from build123d import *

# Parameters (mm, degrees)
BASE_SKETCH_W           = 585.98
BASE_SKETCH_H           = 191.39
BOSS_EXTRUDE1_DEPTH     = 11.81
JOINT_X_W               = 25.4
JOINT_X_H               = 11.81
BOSS_EXTRUDE2_DEPTH     = 11.81
LPATTERN1_COUNT         = 4
LPATTERN1_PITCH         = 186.86
JOINT_Y_W               = 11.81
JOINT_Y_H               = 25.4
BOSS_EXTRUDE3_DEPTH     = 11.81
LPATTERN2_COUNT         = 4
LPATTERN2_PITCH         = 59.266666667
MIRROR3_COPY_1_SKETCH_W = 11.81
MIRROR3_COPY_1_SKETCH_H = 25.4
MIRROR3_COPY_1_DEPTH    = 11.81
MIRROR3_COPY_2_SKETCH_W = 11.81
MIRROR3_COPY_2_SKETCH_H = 25.4
MIRROR3_COPY_2_DEPTH    = 11.81
MIRROR3_COPY_3_SKETCH_W = 11.81
MIRROR3_COPY_3_SKETCH_H = 25.4
MIRROR3_COPY_3_DEPTH    = 11.81


with BuildPart() as part:
    # Base_Sketch → Boss-Extrude1 (new body)
    with BuildSketch(Plane.XY):
        with Locations((0, -4.040082085)):
            Rectangle(BASE_SKETCH_W, BASE_SKETCH_H)
    extrude(amount=BOSS_EXTRUDE1_DEPTH)

    # Joint_X → Boss-Extrude2 (add)
    with BuildSketch(Plane.XY.offset(11.81)):
        with Locations((-280.29, -105.640082085)):
            Rectangle(JOINT_X_W, JOINT_X_H)
    boss_extrude2 = extrude(amount=-BOSS_EXTRUDE2_DEPTH)

    # LPattern1: Boss-Extrude2 ×4
    with Locations(*[(i * LPATTERN1_PITCH, 0, 0) for i in range(1, LPATTERN1_COUNT)]):
        add(boss_extrude2)

    # Joint_Y → Boss-Extrude3 (add)
    with BuildSketch(Plane.XY.offset(11.81)):
        with Locations((-298.895, -98.845082085)):
            Rectangle(JOINT_Y_W, JOINT_Y_H)
    boss_extrude3 = extrude(amount=-BOSS_EXTRUDE3_DEPTH)

    # LPattern2: Boss-Extrude3 ×4
    with Locations(*[(0, i * LPATTERN2_PITCH, 0) for i in range(1, LPATTERN2_COUNT)]):
        add(boss_extrude3)

    # Mirror3: Boss-Extrude3 across plane
    add(boss_extrude3.mirror(Plane.ZY))

    # Mirror3 copy 1 sketch → Mirror3 copy 1 (add)
    with BuildSketch(Plane(origin=(0, 59.266666667, 11.81), x_dir=(-1, 0, 0), z_dir=(0, 0, 1))):
        with Locations((-298.895, 98.845082085)):
            Rectangle(MIRROR3_COPY_1_SKETCH_W, MIRROR3_COPY_1_SKETCH_H)
    extrude(amount=-MIRROR3_COPY_1_DEPTH)

    # Mirror3 copy 2 sketch → Mirror3 copy 2 (add)
    with BuildSketch(Plane(origin=(0, 118.533333333, 11.81), x_dir=(-1, 0, 0), z_dir=(0, 0, 1))):
        with Locations((-298.895, 98.845082085)):
            Rectangle(MIRROR3_COPY_2_SKETCH_W, MIRROR3_COPY_2_SKETCH_H)
    extrude(amount=-MIRROR3_COPY_2_DEPTH)

    # Mirror3 copy 3 sketch → Mirror3 copy 3 (add)
    with BuildSketch(Plane(origin=(0, 177.8, 11.81), x_dir=(-1, 0, 0), z_dir=(0, 0, 1))):
        with Locations((-298.895, 98.845082085)):
            Rectangle(MIRROR3_COPY_3_SKETCH_W, MIRROR3_COPY_3_SKETCH_H)
    extrude(amount=-MIRROR3_COPY_3_DEPTH)


solid = part.part
Can you work these out from the model? Positions are in its coordinate system, mm. A direction names the side the tool comes from. Round coordinates to 2 decimals unless told otherwise and drop trailing zeros. Loops run counter-clockwise (first coordinate to the right, second up) from the corner with the lowest first, then second, coordinate; pieces in that order, holes last. Notation, with made-up numbers: (88.5, 47) - (128.5, 47) arc R33 cw to (128.5, 80) - close; hole circle Ø1 at (69, -11.5). An arc over 180 degrees is marked (long way). Answer in a Markdown table with one row per item. Add a question column.
Q1. For pin 1 Ø12 at (x, y) = (-36.5, 25.5) entering from -Z; pin 2 Ø3.5 at (y, z) = (-5, 4.5) entering from -X; pin 3 Ø3.5 at (y, z) = (-68, 7.5) entering from +X; pin 4 Ø3.5 at (x, z) = (186.5, 4.5) entering from -Y, each with a flat end and sliding along its axis, tell me the tip position at first contact or that it passes through.
Q2. Which directions (+Z, -Z, +X, -X, +Y, -Y) give clear straight access to the entire face, cutting with the end or side of a thin tool? Please do faces 4 (the flat face through (-299, 6.988, 6)), 5 (the flat face through (-304.8, 79, 6)), 6 (the flat face through (292.99, -10, 6)), 7 (the flat face through (267.59, -106, 6)), 8 (the flat face through (304.8, -99, 6)).
Q3. I want a section at B-B on x = 63.5. List the corners of the cut face in (y, z) for me.
Q4. I want a section at A-A on y = -68.5. List the corners of the cut face in (x, z) for me, and give its area (3 significant figures).
Q5. I need wall thicknesses on L1, parallel to Y at x = 132, z = 5.5; L2, parallel to X at y = -75.5, z = 3. Which ranges of each line are inside material? Lowest first, please.
Q6. We'd pull the mould along X, two halves only. Please class faces 1 (the flat face through (304.8, -39, 6)), 2 (the flat face through (-188, -99.735, 6)), 3 (the flat face through (-292.99, -69, 6)): pulls with the +X half, pulls with the -X half, needs draft (parallel to the pull), parting line crosses it, or undercut.
A:
| question | item | result |
|---|---|---|
| 1 | pin 1 | z = 0 |
| 1 | pin 2 | x = -292.99 |
| 1 | pin 3 | x = 292.99 |
| 1 | pin 4 | y = -99.74 |
| 2 | face 4 | +Z, -Z, -X |
| 2 | face 5 | +Z, -Z, -X, +Y, -Y |
| 2 | face 6 | +Z, -Z, +X |
| 2 | face 7 | +Z, -Z, -Y |
| 2 | face 8 | +Z, -Z, +X, +Y, -Y |
| 3 | outline | (-99.74, 0) - (91.65, 0) - (91.65, 11.81) - (-99.74, 11.81) - close |
| 4 | outline | (-292.99, 0) - (292.99, 0) - (292.99, 11.81) - (-292.99, 11.81) - close |
| 4 | area | 6,920 mm^2 |
| 5 | L1 | -99.74 to 91.65 |
| 5 | L2 | -292.99 to 292.99 |
| 6 | face 1 | pulls with the +X half |
| 6 | face 2 | undercut |
| 6 | face 3 | pulls with the -X half |
